from build123d import *

# Parameters (mm, degrees)
SKETCH_1_R          = 4
EXTRUDE_1_DEPTH     = 4
SKETCH_2_R          = 2.5
EXTRUDE_2_DEPTH     = 20
CUT_EXTRUDE_1_DEPTH = 2
CHAMFER_1_SIZE      = 0.2
CHAMFER_2_SIZE      = 0.3


with BuildPart() as part:
    # 草图1 → 凸台-拉伸1 (new body)
    with BuildSketch(Plane(origin=(0, 0, 0), x_dir=(1, 0, 0), z_dir=(0, 1, 0))):
        Circle(SKETCH_1_R)
    extrude(amount=EXTRUDE_1_DEPTH)

    # 草图2 → 凸台-拉伸2 (add)
    with BuildSketch(Plane.XZ):
        Circle(SKETCH_2_R)
    extrude(amount=EXTRUDE_2_DEPTH)

    # 草图11 → 切除-拉伸1 (cut)
    with BuildSketch(Plane(origin=(0, 4, 0), x_dir=(1, 0, 0), z_dir=(0, 1, 0))):
        Polygon((1.154954177, 1.999853541), (-1.154446882, 2.000146427), (-2.309401058, 0.000292887), (-1.154954177, -1.999853541), (1.154446882, -2.000146427), (2.309401058, -0.000292887), align=None)
    extrude(amount=-CUT_EXTRUDE_1_DEPTH, mode=Mode.SUBTRACT)

    # 倒角1
    chamfer_1_edges = [part.edges().sort_by_distance(p)[0] for p in [
        (1.732177617, 4, -0.999780327),
        (0.000253647, 4, -1.999999984),
        (-1.73192397, 4, -1.000219657),
        (-1.732177617, 4, 0.999780327),
        (-0.000253647, 4, 1.999999984),
        (1.73192397, 4, 1.000219657),
        (-4, 4, 0),
    ]]
    chamfer(chamfer_1_edges, length=CHAMFER_1_SIZE)

    # 倒角2
    chamfer_2_edges = [part.edges().sort_by_distance(p)[0] for p in [
        (-2.5, -20, 0),
    ]]
    chamfer(chamfer_2_edges, length=CHAMFER_2_SIZE)


solid = part.part
Geometry check sheet. Reference: the model listing, model coordinates, mm. A direction names the side the tool comes from. Coordinates: 2 decimals unless noted, no trailing zeros. Order: outer loops, then holes, each group sorted by start corner. A loop starts at its lowest first (then second) coordinate and runs counter-clockwise, first axis right, second up. Notation, with made-up numbers: (82.5, 57) -> (114.5, 57) arc R20 cw to (114.5, 79) -> close; hole circle Ø1 at (13, 42). An arc over 180 degrees is marked (long way). Use a Markdown table: item, result. Add a question column.
1. Material ranges on L1, parallel to Y at x = 1.25, z = -1.25; L2, parallel to Y at x = 2.5, z = -0.5; L3, parallel to Z at x = -2, y = -17.5, recorded low to high.
2. Cross-section at A-A (x = 0). Enter the section's corners in (y, z).
3. Set-up check for faces 1 (the face through (0, -20, 0)), 2 (the face through (0, 2, 0)), 3 (the face through (-0.54, -9.71, -2.44)): record each of +Z, -Z, +X, -X, +Y, -Y from which the full face is reachable in a straight line by a thin tool's end or side.
4. Cross-section at B-B (y = -15). Enter the section's corners in (x, z).
5. Go/stop test with flat-tipped pins: pin 1 Ø3 at (x, y) = (2, -14.5) entering from +Z; pin 2 Ø0.5 at (x, y) = (-0.5, 3) entering from +Z; pin 3 Ø4 at (x, y) = (-1, -12) entering from -Z. Record where each tip stops, or that it passes through.
6. Mould release check, pull along X, two halves, no side actions. Record for faces 4 (the face through (2, 4, 2)), 5 (the face through (-0.867, 1.873, 3.905)), 6 (the face through (1.724, 2.913, 1.014)): pulls with the +X half, pulls with the -X half, needs draft (parallel to the pull), parting line crosses it, or undercut.
Filled sheet:
| question | item | result |
|---|---|---|
| 1 | L1 | -20 to 2 |
| 1 | L2 | 0 to 4 |
| 1 | L3 | -1.5 to 1.5 |
| 2 | outline | (-20, -2.2) -> (-19.7, -2.5) -> (0, -2.5) -> (0, -4) -> (3.8, -4) -> (4, -3.8) -> (4, -2.2) -> (3.8, -2) -> (2, -2) -> (2, 2) -> (3.8, 2) -> (4, 2.2) -> (4, 3.8) -> (3.8, 4) -> (0, 4) -> (0, 2.5) -> (-19.7, 2.5) -> (-20, 2.2) -> close |
| 3 | face 1 | +Z, -Z, +X, -X, -Y |
| 3 | face 2 | +Y |
| 3 | face 3 | -Y |
| 4 | outline | circle Ø5 at (0, 0) |
| 5 | pin 1 | z = 2.45 |
| 5 | pin 2 | z = 3.99 |
| 5 | pin 3 | z = -2.5 |
| 6 | face 4 | needs draft |
| 6 | face 5 | parting line crosses it |
| 6 | face 6 | undercut |
